```python
from build123d import *

# Parameters (mm, degrees)
SKETCH1_W                                       = 40.4
SKETCH1_H                                       = 12
BOSS_EXTRUDE1_DEPTH                             = 22
CUT_EXTRUDE1_REACH                              = 34.188
SKETCH2_W                                       = 31.5
SKETCH2_H                                       = 20
CUT_EXTRUDE2_REACH                              = 48.391
SKETCH4_R                                       = 0.9
CHAMFER1_SIZE                                   = 3.5
CSK_FOR_M2_FLAT_HEAD_MACHINE_SCREW1_D           = 2.4
CSK_FOR_M2_FLAT_HEAD_MACHINE_SCREW1_DEPTH       = 12.7
CSK_FOR_M2_FLAT_HEAD_MACHINE_SCREW1_CSINK_D     = 4.4
CSK_FOR_M2_FLAT_HEAD_MACHINE_SCREW1_CSINK_ANGLE = 90
CSK_FOR_M2_FLAT_HEAD_MACHINE_SCREW1_TIP         = 0.721032743
CHAMFER2_SIZE                                   = 4
BOSS_EXTRUDE2_START                             = 0.5
SKETCH20_R                                      = 2.5
SKETCH20_R_2                                    = 1.2
BOSS_EXTRUDE2_DEPTH                             = 0.5
BOSS_EXTRUDE3_DEPTH                             = 12
CUT_EXTRUDE3_DEPTH                              = 2.4
SKETCH23_R                                      = 3.65
CUT_EXTRUDE4_DEPTH                              = 22.4
SKETCH24_W                                      = 5.5
SKETCH24_H                                      = 5.5
CUT_EXTRUDE5_DEPTH                              = 22.4
SKETCH26_W                                      = 10
SKETCH26_H                                      = 5
BOSS_EXTRUDE4_DEPTH                             = 11.375
SKETCH27_W                                      = 10
SKETCH27_H                                      = 25
BOSS_EXTRUDE5_DEPTH                             = 6.5
CUT_EXTRUDE6_DEPTH                              = 2.4
SKETCH29_R                                      = 3.35
CUT_EXTRUDE7_DEPTH                              = 54.60028568
CHAMFER3_SIZE                                   = 2
CHAMFER5_SIZE                                   = 2
CHAMFER6_SIZE                                   = 4.5


with BuildPart() as part:
    # Sketch1 → Boss-Extrude1 (new body)
    with BuildSketch(Plane.XY):
        Rectangle(SKETCH1_W, SKETCH1_H)
    extrude(amount=BOSS_EXTRUDE1_DEPTH)

    # Sketch2 → Cut-Extrude1 (cut, up to next)
    with BuildSketch(Plane(origin=(0, 6, 0), x_dir=(1, 0, 0), z_dir=(0, 1, 0)), mode=Mode.PRIVATE) as cut_extrude1_sk1:
        with Locations((1.85, -10)):
            Rectangle(SKETCH2_W, SKETCH2_H)
    cut_extrude1_tool1 = extrude(cut_extrude1_sk1.sketch, amount=-CUT_EXTRUDE1_REACH, mode=Mode.PRIVATE) & part.part
    add(cut_extrude1_tool1.solids().sort_by_distance((1.85, 6, 10))[0], mode=Mode.SUBTRACT)

    # Sketch4 → Cut-Extrude2 (cut, up to next)
    with BuildSketch(Plane(origin=(20.2, 0, 0), x_dir=(0, 0, -1), z_dir=(1, 0, 0)), mode=Mode.PRIVATE) as cut_extrude2_sk1:
        with Locations((-6, 0)):
            Circle(SKETCH4_R)
    cut_extrude2_tool1 = extrude(cut_extrude2_sk1.sketch, amount=-CUT_EXTRUDE2_REACH, mode=Mode.PRIVATE) & part.part
    add(cut_extrude2_tool1.solids().sort_by_distance((20.2, 0, 6))[0], mode=Mode.SUBTRACT)

    # Chamfer1
    chamfer1_edges = [part.edges().sort_by_distance(p)[0] for p in [
        (-17.05, -6, 0),
        (-17.05, 6, 0),
        (18.9, -6, 0),
        (18.9, 6, 0),
    ]]
    chamfer(chamfer1_edges, length=CHAMFER1_SIZE)

    # CSK for M2 Flat Head Machine Screw1
    with Locations(Plane(origin=(20.2, 0, 0), x_dir=(0, 0, -1), z_dir=(1, 0, 0))):
        with Locations((-6, 0)):
            CounterSinkHole(CSK_FOR_M2_FLAT_HEAD_MACHINE_SCREW1_D / 2, CSK_FOR_M2_FLAT_HEAD_MACHINE_SCREW1_CSINK_D / 2, depth=CSK_FOR_M2_FLAT_HEAD_MACHINE_SCREW1_DEPTH, counter_sink_angle=CSK_FOR_M2_FLAT_HEAD_MACHINE_SCREW1_CSINK_ANGLE)
            with Locations((0, 0, -(CSK_FOR_M2_FLAT_HEAD_MACHINE_SCREW1_DEPTH + CSK_FOR_M2_FLAT_HEAD_MACHINE_SCREW1_TIP / 2))):  # 118° drill point
                Cone(0, CSK_FOR_M2_FLAT_HEAD_MACHINE_SCREW1_D / 2, CSK_FOR_M2_FLAT_HEAD_MACHINE_SCREW1_TIP, mode=Mode.SUBTRACT)

    # Chamfer2
    # the kernel refuses this chamfer: 4 mm, written as the material it takes off along each edge
    with BuildSketch(Plane(origin=(20.2, 12.786731952, 0), x_dir=(-0.9996219169112968, 0, -0.027495876610586365), z_dir=(0, -1, 0))) as chamfer2_piece_1:
        Polygon((CHAMFER2_SIZE * 0.999621916911, -CHAMFER2_SIZE * 0.0274958766106), (-CHAMFER2_SIZE * 0.0274958766106, -CHAMFER2_SIZE * 0.999621916911), (0, 0), align=None)
    extrude(amount=25.573463904, mode=Mode.SUBTRACT)

    # Sketch20 → Boss-Extrude2 (add)
    with BuildSketch(Plane.ZY.offset(-17.6).offset(BOSS_EXTRUDE2_START)):
        with Locations(Location((6, 0, 0), (0, 0, 180))):
            Circle(SKETCH20_R)
        with Locations(Location((6, 0, 0), (0, 0, 180))):
            Circle(SKETCH20_R_2, mode=Mode.SUBTRACT)
    extrude(amount=-BOSS_EXTRUDE2_DEPTH)

    # Sketch25 → Boss-Extrude3 (add, through all)
    with BuildSketch(Plane.XZ.offset(6)):
        Polygon((20.2, 22), (-20.2, 22), (-5, 25), (5, 25), align=None)
    extrude(amount=-BOSS_EXTRUDE3_DEPTH)

    # Sketch5 → Cut-Extrude3 (cut)
    with BuildSketch(Plane.ZY.offset(20.2)):
        with BuildLine():
            Line((6.343920973, 3.633760912), (22.64787234, 2.090656963))
            ThreePointArc((22.64787234, 2.090656963), (24.55, 0), (22.64787234, -2.090656963))
            Line((22.64787234, -2.090656963), (6.343920973, -3.633760912))
            ThreePointArc((6.343920973, -3.633760912), (2.35, 0), (6.343920973, 3.633760912))
        make_face()
    extrude(amount=-CUT_EXTRUDE3_DEPTH, mode=Mode.SUBTRACT)

    # Sketch23 → Cut-Extrude4 (cut)
    with BuildSketch(Plane.ZY.offset(17.8)):
        with Locations((6, 0)):
            Circle(SKETCH23_R)
    extrude(amount=-CUT_EXTRUDE4_DEPTH, mode=Mode.SUBTRACT)

    # Sketch24 → Cut-Extrude5 (cut)
    with BuildSketch(Plane(origin=(0, 0, 0), x_dir=(-1, 0, 0), z_dir=(0, -1, 0))):
        with Locations((13.9, -6)):
            Rectangle(SKETCH24_W, SKETCH24_H)
    extrude(amount=CUT_EXTRUDE5_DEPTH, mode=Mode.SUBTRACT)

    # Sketch26 → Boss-Extrude4 (add)
    with BuildSketch(Plane(origin=(0, -6, 0), x_dir=(1, 0, 0), z_dir=(0, 1, 0))):
        with Locations((0, -22.5)):
            Rectangle(SKETCH26_W, SKETCH26_H)
    extrude(amount=-BOSS_EXTRUDE4_DEPTH)

    # Sketch27 → Boss-Extrude5 (add)
    with BuildSketch(Plane(origin=(0, -17.375, 0), x_dir=(-1, 0, 0), z_dir=(0, -1, 0))):
        with Locations((0, -32.5)):
            Rectangle(SKETCH27_W, SKETCH27_H)
    extrude(amount=-BOSS_EXTRUDE5_DEPTH)

    # Sketch28 → Cut-Extrude6 (cut)
    with BuildSketch(Plane(origin=(0, -17.375, 0), x_dir=(-1, 0, 0), z_dir=(0, -1, 0))):
        with BuildLine():
            Line((-1.791991683, -23.380395137), (-3.335095631, -39.684346505))
            ThreePointArc((-3.335095631, -39.684346505), (0, -43.35), (3.335095631, -39.684346505))
            Line((3.335095631, -39.684346505), (1.791991683, -23.380395137))
            ThreePointArc((1.791991683, -23.380395137), (0, -21.75), (-1.791991683, -23.380395137))
        make_face()
    extrude(amount=-CUT_EXTRUDE6_DEPTH, mode=Mode.SUBTRACT)

    # Sketch29 → Cut-Extrude7 (cut, through all)
    with BuildSketch(Plane(origin=(0, -14.975, 0), x_dir=(-1, 0, 0), z_dir=(0, -1, 0))):
        with Locations(Location((0, -40, 0), (0, 0, 174.593288878))):
            Circle(SKETCH29_R)
    extrude(amount=-CUT_EXTRUDE7_DEPTH, mode=Mode.SUBTRACT)

    # Chamfer3
    # the kernel refuses this chamfer: 2 mm, written as the material it takes off along each edge
    with BuildSketch(Plane(origin=(10.143365976, -17.375, 20), x_dir=(0, 0.9996219169112968, -0.0274958766105856), z_dir=(-1, 0, 0))) as chamfer3_piece_1:
        Polygon((CHAMFER3_SIZE * 0.999621916911, -CHAMFER3_SIZE * 0.0274958766106), (-CHAMFER3_SIZE * 0.0274958766106, -CHAMFER3_SIZE * 0.999621916911), (0, 0), align=None)
    extrude(amount=20.286731952, mode=Mode.SUBTRACT)
    with BuildSketch(Plane(origin=(-5, -22.518365976, 45), x_dir=(-0.02749587661058651, 0, -0.9996219169112968), z_dir=(0, 1, 0))) as chamfer3_piece_2:
        Polygon((CHAMFER3_SIZE * 0.999621916911, -CHAMFER3_SIZE * 0.0274958766106), (-CHAMFER3_SIZE * 0.0274958766106, -CHAMFER3_SIZE * 0.999621916911), (0, 0), align=None)
    extrude(amount=16.786731952, mode=Mode.SUBTRACT)
    with BuildSketch(Plane(origin=(5, -22.518365976, 45), x_dir=(0.02749587661058651, 0, -0.9996219169112968), z_dir=(0, 1, 0))) as chamfer3_piece_3:
        Polygon((CHAMFER3_SIZE * 0.999621916911, CHAMFER3_SIZE * 0.0274958766106), (-CHAMFER3_SIZE * 0.0274958766106, CHAMFER3_SIZE * 0.999621916911), (0, 0), align=None)
    extrude(amount=16.786731952, mode=Mode.SUBTRACT)

    # Chamfer5
    chamfer5_edges = [part.edges().sort_by_distance(p)[0] for p in [
        (0, -10.875, 25),
    ]]
    chamfer(chamfer5_edges, length=CHAMFER5_SIZE)

    # Chamfer6
    # the kernel refuses this chamfer: 4.5 mm, written as the material it adds along each edge
    with BuildSketch(Plane(origin=(-5, -6, 20), x_dir=(0.027495876610586587, -0.9996219169112966, 0), z_dir=(0, 0, 1))) as chamfer6_piece_1_section:
        Polygon((CHAMFER6_SIZE * 0.999621916911, -CHAMFER6_SIZE * 0.0274958766106), (-CHAMFER6_SIZE * 0.0274958766106, -CHAMFER6_SIZE * 0.999621916911), (0, 0), align=None)
    chamfer6_piece_1 = extrude(amount=16.572573446, mode=Mode.PRIVATE)
    chamfer6_piece_1 = split(chamfer6_piece_1, bisect_by=Plane(origin=(-6.365694547, -6.762864523, 22.887864523), z_dir=(0, -0.7071067811865476, -0.7071067811865476)), keep=Keep.TOP, mode=Mode.PRIVATE)
    add(chamfer6_piece_1)
    with BuildSketch(Plane(origin=(-5, -6, 20), x_dir=(0.027495876610586587, -0.9996219169112966, 0), z_dir=(0, 0, 1))) as chamfer6_piece_2_section:
        Polygon((CHAMFER6_SIZE * 0.999621916911, -CHAMFER6_SIZE * 0.0274958766106), (-CHAMFER6_SIZE * 0.0274958766106, -CHAMFER6_SIZE * 0.999621916911), (0, 0), align=None)
    chamfer6_piece_2 = extrude(amount=16.572573446, mode=Mode.PRIVATE)
    chamfer6_piece_2 = split(chamfer6_piece_2, bisect_by=Plane(origin=(-6.882801267, -6.788517358, 24.628394487), z_dir=(0.19363303189666034, 0, -0.9810740282764124)), keep=Keep.TOP, mode=Mode.PRIVATE)
    add(chamfer6_piece_2)
    with BuildSketch(Plane(origin=(5, -6, 36.572573446), x_dir=(-0.0274958766105862, -0.9996219169112969, 0), z_dir=(0, 0, -1))) as chamfer6_piece_3_section:
        Polygon((CHAMFER6_SIZE * 0.999621916911, -CHAMFER6_SIZE * 0.0274958766106), (-CHAMFER6_SIZE * 0.0274958766106, -CHAMFER6_SIZE * 0.999621916911), (0, 0), align=None)
    chamfer6_piece_3 = extrude(amount=16.572573446, mode=Mode.PRIVATE)
    chamfer6_piece_3 = split(chamfer6_piece_3, bisect_by=Plane(origin=(5.40625, -9.484375, 25.609375), z_dir=(0, -0.7071067811865476, -0.7071067811865476)), keep=Keep.TOP, mode=Mode.PRIVATE)
    add(chamfer6_piece_3)
    with BuildSketch(Plane(origin=(5, -6, 36.572573446), x_dir=(-0.0274958766105862, -0.9996219169112969, 0), z_dir=(0, 0, -1))) as chamfer6_piece_4_section:
        Polygon((CHAMFER6_SIZE * 0.999621916911, -CHAMFER6_SIZE * 0.0274958766106), (-CHAMFER6_SIZE * 0.0274958766106, -CHAMFER6_SIZE * 0.999621916911), (0, 0), align=None)
    chamfer6_piece_4 = extrude(amount=16.572573446, mode=Mode.PRIVATE)
    chamfer6_piece_4 = split(chamfer6_piece_4, bisect_by=Plane(origin=(6.882801267, -6.788517358, 24.628394487), z_dir=(-0.19363303189666034, 0, -0.9810740282764124)), keep=Keep.TOP, mode=Mode.PRIVATE)
    add(chamfer6_piece_4)


solid = part.part
```
Verification items for the finished model (mm, model axes). A direction names the side the tool comes from. Give positions to 0.01 mm unless a question says otherwise; leave off trailing zeros. Order: outer loops, then holes, each group sorted by start corner. A loop starts at its lowest first (then second) coordinate and runs counter-clockwise, first axis right, second up. Notation, with made-up numbers: (-23.75, -4) - (13.25, -4) arc R27 ccw to (13.25, 20) - close; hole circle Ø4 at (29.5, 27). An arc over 180 degrees is marked (long way). Answer as CSV lines item,"result". Start each with the question number.
Item 1: Material ranges on L1, parallel to X at y = -16.4, z = 40; L2, parallel to Y at x = -18.3, z = 6; L3, parallel to Z at x = -14.75, y = 0, recorded low to high.
Item 2: Mould release check, pull along X, two halves, no side actions. Record for faces 1 (the face through (0.07, -16.361, 20.986)), 2 (the face through (-15, -4, 3.25)), 3 (the face through (-4, -14, 44)): released by +X, released by -X, zero draft, split by the parting line, or undercut.
Item 3: Section check B-B, the plane z = 12. Record the boundary of the cut face in (x, y).
Item 4: Access from +Z, -Z, +X, -X, +Y, -Y to the whole of each face (thin tool, end or side, straight path). Record for faces 4 (the face through (-2.574, -16.192, 31.646)), 5 (the face through (18, -6, 15)), 6 (the face through (0, -1, 25)), 7 (the face through (-19.02, -2.86, 14.52)), 8 (the face through (-13.9, 0, 12)).
Item 5: Gauge pin test, flat ends, axial feed: pin 1 (2 mm diameter, centred on x = -15.5, y = -5, fed in from -Z); pin 2 (2.5 mm diameter, centred on y = 1, z = 5.5, fed in from -X); pin 3 (1.4 mm diameter, centred on y = 0, z = 6, fed in from +X); pin 4 (6 mm diameter, centred on y = -11.5, z = 29.5, fed in from +X). Record the tip position at first contact, or that the pin passes through.
Item 6: Section check C-C, the plane y = -11.5. Record the boundary of the cut face in (x, z), plus the area to 3 significant figures.
Item 7: Section check D-D, the plane x = 0. Record the boundary of the cut face in (y, z) (3 decimals), plus the area to 3 significant figures.
Item 8: Section check A-A, the plane y = 0. Record the boundary of the cut face in (x, z).
Filled in:
1,L1,"-5 to -3.35, 3.35 to 5"
1,L2,"-6 to -3.65, 3.65 to 6"
1,L3,"0 to 2.35, 9.65 to 23.08"
2,face 1,"zero draft"
2,face 2,"undercut"
2,face 3,"released by -X"
3,outline,"(-20.2, -6) - (-13.9, -6) - (-13.9, 6) - (-20.2, 6) - (-20.2, 3.1) - (-17.8, 3.1) - (-17.8, -3.1) - (-20.2, -3.1) - close; (17.6, -6) - (20.2, -6) - (20.2, 6) - (17.6, 6) - close"
4,face 4,"-Y"
4,face 5,"+Z, -Z, +X, -Y"
4,face 6,"+Z, +X, -X, +Y"
4,face 7,"-X"
4,face 8,"-Z, +Y, -Y"
5,pin 1,"z = 1.5"
5,pin 2,"x = 17.1"
5,pin 3,"through"
5,pin 4,"x = 5"
6,outline,"(-5, 20) - (5, 20) - (5, 43) - (3, 45) - (-3, 45) - (-5, 43) - close; hole circle Ø6.7 at (0, 40)"
6,area,"211 mm^2"
7,outline,"(-17.375, 43.35) - (-10.875, 43.35) - (-10.875, 45) - (-17.375, 45) - close; (-17.125, 21.75) - (-15.375, 20) - (6, 20) - (6, 25) - (-8.875, 25) - (-10.875, 27) - (-10.875, 36.65) - (-14.975, 36.65) - (-14.975, 21.75) - close"
7,area,"168 mm^2"
8,outline,"(-20.2, 0) - (-13.9, 0) - (-13.9, 2.35) - (-20.2, 2.35) - close; (-17.8, 9.65) - (-13.9, 9.65) - (-13.9, 20) - (17.6, 20) - (17.6, 8.5) - (17.1, 8.5) - (17.1, 7.2) - (19.2, 7.2) - (20.2, 8.2) - (20.2, 22) - (5, 25) - (-5, 25) - (-17.8, 22.47) - close; (17.1, 3.5) - (17.6, 3.5) - (17.6, 1.4) - (20.1, 3.9) - (19.2, 4.8) - (17.1, 4.8) - close"
